from build123d import *

# Parameters (mm, degrees)
SKETCH1_R                 = 3.175
BOSS_EXTRUDE1_DEPTH       = 63.5
M3X0_5_TAPPED_HOLE1_D     = 2.5
M3X0_5_TAPPED_HOLE1_DEPTH = 12.7
M3X0_5_TAPPED_HOLE1_TIP   = 0.751075774
M3X0_5_TAPPED_HOLE2_D     = 2.5
M3X0_5_TAPPED_HOLE2_DEPTH = 12.7
M3X0_5_TAPPED_HOLE2_TIP   = 0.751075774


with BuildPart() as part:
    # Sketch1 → Boss-Extrude1 (new body)
    with BuildSketch(Plane(origin=(0, 0, 0), x_dir=(1, 0, 0), z_dir=(0, 1, 0))):
        Circle(SKETCH1_R)
    extrude(amount=BOSS_EXTRUDE1_DEPTH)

    # M3x0.5 Tapped Hole1
    with Locations(Plane(origin=(0, 63.5, 0), x_dir=(1, 0, 0), z_dir=(0, 1, 0))):
        with Locations((0, 0)):
            Hole(M3X0_5_TAPPED_HOLE1_D / 2, depth=M3X0_5_TAPPED_HOLE1_DEPTH)
            with Locations((0, 0, -(M3X0_5_TAPPED_HOLE1_DEPTH + M3X0_5_TAPPED_HOLE1_TIP / 2))):  # 118° drill point
                Cone(0, M3X0_5_TAPPED_HOLE1_D / 2, M3X0_5_TAPPED_HOLE1_TIP, mode=Mode.SUBTRACT)

    # M3x0.5 Tapped Hole2
    with Locations(Plane(origin=(0, 0, 0), x_dir=(-1, 0, 0), z_dir=(0, -1, 0))):
        with Locations((0, 0)):
            Hole(M3X0_5_TAPPED_HOLE2_D / 2, depth=M3X0_5_TAPPED_HOLE2_DEPTH)
            with Locations((0, 0, -(M3X0_5_TAPPED_HOLE2_DEPTH + M3X0_5_TAPPED_HOLE2_TIP / 2))):  # 118° drill point
                Cone(0, M3X0_5_TAPPED_HOLE2_D / 2, M3X0_5_TAPPED_HOLE2_TIP, mode=Mode.SUBTRACT)


solid = part.part
CAD build for the part. Positions are in the model's coordinates, mm. A direction names the side the tool comes from. Give positions to 0.01 mm unless a question says otherwise; leave off trailing zeros. Loops run counter-clockwise (first coordinate to the right, second up) from the corner with the lowest first, then second, coordinate; pieces in that order, holes last. Notation, with made-up numbers: M 23,38.5 L 67,38.5 A6 ccw 67,46.5 Z; hole C 76,-20 d2. An arc over 180 degrees is marked long. One line per question, with ' | ' between items. Start each with the question number.
1. Saw through at B-B on z = 2. Give the cut face in (x, y).
2. Saw through at A-A on y = 30. Give the cut face in (x, z) (3 decimals), plus the area to 3 significant figures.
3. 3-axis set-ups, long thin cutter, end or side, ignore diameter. For faces 1 (the face through (0.27, 57.06, 1.22)), 2 (the face through (1, 0, 1)): which of +Z, -Z, +X, -X, +Y, -Y reach the whole face in a straight line?
4. Two-plate mould, pull along Z, no slides. Class faces 3 (the face through (-0.27, 6.44, 1.22)), 4 (the face through (1, 63.5, 1)), 5 (the face through (-0.69, 31.31, 3.1)): pulls with the +Z half, pulls with the -Z half, needs draft (parallel to the pull), parting line crosses it, or undercut.
5. Probe L1, parallel to Z at x = 0, y = 55.5 (3 decimals); L2, parallel to X at y = 21.5, z = -0.25; L3, parallel to X at y = 53.5, z = 1.75. List the from-to ranges inside material, lowest first. Write a range as from..to.
6. Flat gauge pins, fed straight in: pin 1 (3 mm diameter, centred on y = 22, z = -1.5, fed in from -X) (3 decimals); pin 2 (1.5 mm diameter, centred on x = -1, y = 36, fed in from +Z); pin 3 (2 mm diameter, centred on x = 0, z = 0, fed in from +Y). Where does each tip first touch, or does it go through?
7. Saw through at C-C on x = 2.5. Give the cut face in (y, z), plus the area to 3 significant figures.
Result sheet:
1) outline: M -2.47,0 L 2.47,0 L 2.47,63.5 L -2.47,63.5 Z
2) outline: C 0,0 d6.35 | area: 31.7 mm^2
3) face 1: +Y | face 2: +Z, -Z, +X, -X, -Y
4) face 3: undercut | face 4: needs draft | face 5: parting line crosses it
5) L1: z = -3.175..-1.25, 1.25..3.175 | L2: x = -3.17..3.17 | L3: x = -2.65..2.65
6) pin 1: stops at x = -3.175 | pin 2: stops at z = 3.17 | pin 3: stops at y = 50.65
7) outline: M 0,-1.96 L 63.5,-1.96 L 63.5,1.96 L 0,1.96 Z | area: 249 mm^2
